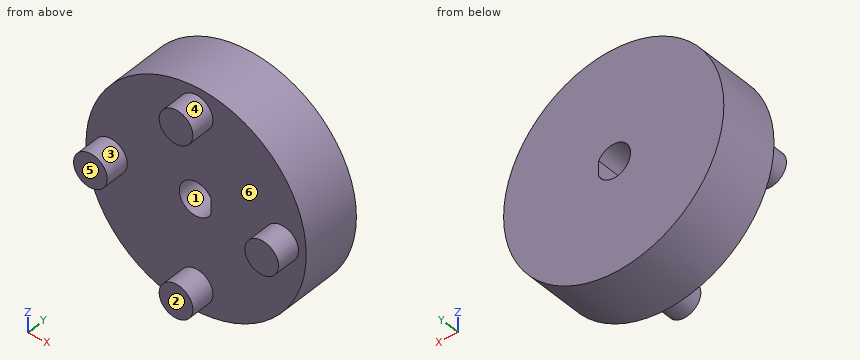
```python
from build123d import *

# Parameters (mm, degrees)
F0_R     = 9
F0_R_2   = 1.375
F0_R_3   = 4
F1_DEPTH = 2
F2_DEPTH = 4
F3_DEPTH = 3


with BuildPart() as f1:
    # F0 (on Front) → F1 (new body)
    with BuildSketch(Plane.XZ):
        Circle(F0_R)
        with Locations((0, -7)):
            Circle(F0_R_2, mode=Mode.SUBTRACT)
        with Locations((-7, 0)):
            Circle(F0_R_2, mode=Mode.SUBTRACT)
        Circle(F0_R_3, mode=Mode.SUBTRACT)
        with Locations((7, 0)):
            Circle(F0_R_2, mode=Mode.SUBTRACT)
        with Locations((0, 7)):
            Circle(F0_R_2, mode=Mode.SUBTRACT)
        Circle(F0_R_3)
        with BuildLine():
            ThreePointArc((1.2252600864, 0.6239893595), (1.337041065, 0.3208522879), (1.375, 0))
            ThreePointArc((1.375, 0), (1.337041065, -0.3208522879), (1.2252600864, -0.6239893595))
            ThreePointArc((1.2252600864, -0.6239893595), (-1.375, 0), (1.2252600864, 0.6239893595))
        make_face(mode=Mode.SUBTRACT)
        with Locations((0, 7)):
            Circle(F0_R_2)
        with BuildLine():
            ThreePointArc((1.2252600864, -0.6239893595), (1.337041065, -0.3208522879), (1.375, 0))
            ThreePointArc((1.375, 0), (1.337041065, 0.3208522879), (1.2252600864, 0.6239893595))
            Line((1.2252600864, 0.6239893595), (1.2252600864, -0.6239893595))
        make_face()
    extrude(amount=F1_DEPTH)

    # F0 (on Front) → F2 (join)
    with BuildSketch(Plane.XZ):
        with Locations((-7, 0)):
            Circle(F0_R_2)
        with Locations((0, 7)):
            Circle(F0_R_2)
        with Locations((7, 0)):
            Circle(F0_R_2)
        with Locations((0, -7)):
            Circle(F0_R_2)
    extrude(amount=F2_DEPTH)

    # F0 (on Front) → F3 (join)
    with BuildSketch(Plane.XZ):
        Circle(F0_R)
        with Locations((0, -7)):
            Circle(F0_R_2, mode=Mode.SUBTRACT)
        with Locations((-7, 0)):
            Circle(F0_R_2, mode=Mode.SUBTRACT)
        Circle(F0_R_3, mode=Mode.SUBTRACT)
        with Locations((7, 0)):
            Circle(F0_R_2, mode=Mode.SUBTRACT)
        with Locations((0, 7)):
            Circle(F0_R_2, mode=Mode.SUBTRACT)
        Circle(F0_R_3)
        with BuildLine():
            ThreePointArc((1.2252600864, 0.6239893595), (1.337041065, 0.3208522879), (1.375, 0))
            ThreePointArc((1.375, 0), (1.337041065, -0.3208522879), (1.2252600864, -0.6239893595))
            ThreePointArc((1.2252600864, -0.6239893595), (-1.375, 0), (1.2252600864, 0.6239893595))
        make_face(mode=Mode.SUBTRACT)
        with Locations((7, 0)):
            Circle(F0_R_2)
        with Locations((0, 7)):
            Circle(F0_R_2)
        with Locations((-7, 0)):
            Circle(F0_R_2)
        with Locations((0, -7)):
            Circle(F0_R_2)
        with BuildLine():
            ThreePointArc((1.2252600864, -0.6239893595), (1.337041065, -0.3208522879), (1.375, 0))
            ThreePointArc((1.375, 0), (1.337041065, 0.3208522879), (1.2252600864, 0.6239893595))
            Line((1.2252600864, 0.6239893595), (1.2252600864, -0.6239893595))
        make_face()
    extrude(amount=-F3_DEPTH)


solid = f1.part
```
Can you work these out from the model? Positions are in its coordinate system, mm. Face numbers are marked on the shaded views. A direction names the side the tool comes from. Round coordinates to 2 decimals unless told otherwise and drop trailing zeros. Loops run counter-clockwise (first coordinate to the right, second up) from the corner with the lowest first, then second, coordinate; pieces in that order, holes last. Notation, with made-up numbers: M 85,-18 L 114,-18 A22 cw 114,21 Z; hole C 58,-14 d5. An arc over 180 degrees is marked long. Answer as a JSON object with one key per item and string values. Group by question number.
Q1. Imagine slicing it at D-D, the plane z = 3. Please give me the cut outline in (x, y), then the cut area to 3 significant figures.
Q2. Imagine slicing it at B-B, the plane z = -7.25. Please give me the cut outline in (x, y), then the cut area to 3 significant figures.
Q3. Please list where these lines run through material, in increasing order: L1, parallel to Z at x = 0, y = -0.65 (3 decimals); L2, parallel to Y at x = -5.75, z = -1; L3, parallel to Z at x = -0.75, y = -1.5.
Q4. On a 3-axis mill with a long thin cutter (end or side, diameter ignored), from which of +Z, -Z, +X, -X, +Y, -Y can I reach the whole of each face in a straight line? I mean the marked faces 5 and 6. Say none if no direction works.
Q5. Imagine slicing it at A-A, the plane x = 0. Please give me the cut outline in (y, z) (3 decimals).
Q6. Imagine slicing it at C-C, the plane x = -7. Please give me the cut outline in (y, z) (3 decimals), then the cut area to 3 significant figures.
Q7. We'd pull the mould along X, two halves only. Please class the marked faces 1, 2, 3 and 4: +X half, -X half, draft (parallel to the pull), parting line (faces both ways), or undercut.
Q8. Will these pins go through, and if not, where does the flat tip stop? pin 1 (4 mm diameter, centred on x = 3.5, y = -0.5, fed in from -Z); pin 2 (2 mm diameter, centred on y = -2, z = 1.5, fed in from +X); pin 3 (3 mm diameter, centred on x = -5, y = 1, fed in from +Z); pin 4 (2 mm diameter, centred on x = 0, z = 0, fed in from -Y).
Findings:
{
 "1": {"outline": "M -8.49,-2 L 8.49,-2 L 8.49,3 L -8.49,3 Z", "area": "84.9 mm2"},
 "2": {"outline": "M -5.33,-2 L -1.35,-2 L -1.35,-4 L 1.35,-4 L 1.35,-2 L 5.33,-2 L 5.33,3 L -5.33,3 Z", "area": "58.7 mm2"},
 "3": {"L1": "z = -9 to -1.375, 1.375 to 9", "L2": "y = -2 to 3", "L3": "z = -8.97 to -1.15, 1.15 to 8.97"},
 "4": {"face 5": "+Z, -Z, +X, -X, -Y", "face 6": "-Y"},
 "5": {"outline": "M -4,-8.375 L -2,-8.375 L -2,-9 L 3,-9 L 3,-1.375 L -2,-1.375 L -2,-5.625 L -4,-5.625 Z; M -4,5.625 L -2,5.625 L -2,1.375 L 3,1.375 L 3,9 L -2,9 L -2,8.375 L -4,8.375 Z"},
 "6": {"outline": "M -4,-1.375 L -2,-1.375 L -2,-5.657 L 3,-5.657 L 3,5.657 L -2,5.657 L -2,1.375 L -4,1.375 Z", "area": "62.1 mm2"},
 "7": {"face 1": "undercut", "face 2": "draft", "face 3": "undercut", "face 4": "parting line"},
 "8": {"pin 1": "stops at z = -8.87", "pin 2": "stops at x = 8.99", "pin 3": "stops at z = 8.29", "pin 4": "passes through"}
}
